The model under review builds one solid part; all positions refer to its coordinate system, in mm. A direction names the side the tool comes from. Coordinates: 2 decimals unless noted, no trailing zeros. Loops run counter-clockwise (first coordinate to the right, second up) from the corner with the lowest first, then second, coordinate; pieces in that order, holes last. Notation, with made-up numbers: M 66.25,33.5 L 125.25,33.5 A16 cw 125.25,51.5 Z; hole C 28.25,85.25 d4. An arc over 180 degrees is marked long. Return JSON: item names as keys, results as strings.
```python
from build123d import *

# Parameters (mm, degrees)
PAD_DEPTH       = 10.5
CHAMFER001_SIZE = 1
SKETCH017_R     = 1.6
POCKET010_DEPTH = 12
SKETCH018_R     = 1.95
POCKET011_DEPTH = 5
FILLET001_R     = 5
CHAMFER002_SIZE = 1
CHAMFER003_SIZE = 2.5


with BuildPart() as part:
    # Sketch016 → Pad (new body)
    with BuildSketch(Plane.XY):
        with BuildLine():
            Line((-12.5, 0), (-12.5, 10.25))
            Line((-12.5, 10.25), (-25.5, 10.25))
            Line((-25.5, 10.25), (-25.5, -26))
            Line((-25.5, -26), (25.3, -26))
            ThreePointArc((25.3, -26), (38.735029, -20.435029), (44.3, -7))
            Line((44.3, -7), (25.3, -7))
            Line((25.3, -7), (25.3, -12.5))
            Line((25.3, -12.5), (0, -12.5))
            ThreePointArc((-12.5, 0), (-8.838835, -8.838835), (0, -12.5))
        make_face()
    extrude(amount=PAD_DEPTH)

    # Chamfer001
    chamfer001_edges = [part.edges().sort_by_distance(p)[0] for p in [
        (44.3, -7, 5.25),
    ]]
    chamfer(chamfer001_edges, length=CHAMFER001_SIZE)

    # Sketch017 (on Face7 of Chamfer001) → Pocket010 (cut)
    with BuildSketch(Plane(origin=(-25.5, 0, 0), x_dir=(0, -1, 0), z_dir=(-1, 0, 0))):
        with Locations((-5.75, 3.7)):
            Circle(SKETCH017_R)
        with Locations((21.5, 3.7)):
            Circle(SKETCH017_R)
    extrude(amount=-POCKET010_DEPTH, mode=Mode.SUBTRACT)

    # Sketch018 (on Face7 of Pocket010) → Pocket011 (cut)
    with BuildSketch(Plane(origin=(-25.5, 0, 0), x_dir=(0, -1, 0), z_dir=(-1, 0, 0))):
        with Locations((-5.75, 3.7)):
            Circle(SKETCH018_R)
        with Locations((21.5, 3.7)):
            Circle(SKETCH018_R)
    extrude(amount=-POCKET011_DEPTH, mode=Mode.SUBTRACT)

    # Fillet001
    fillet001_edges = [part.edges().sort_by_distance(p)[0] for p in [
        (-12.5, 10.25, 5.25),
    ]]
    fillet(fillet001_edges, radius=FILLET001_R)

    # Chamfer002
    chamfer002_edges = [part.edges().sort_by_distance(p)[0] for p in [
        (-21.5, 10.25, 10.5),
        (-0.1, -26, 10.5),
        (-13.964466, 8.785534, 10.5),
        (-12.5, 2.625, 10.5),
        (-8.838835, -8.838835, 10.5),
        (38.376823, -20.783929, 10.5),
        (43.786842, -7.499827, 10.5),
        (34.3, -7, 10.5),
        (25.3, -9.75, 10.5),
        (12.65, -12.5, 10.5),
    ]]
    chamfer(chamfer002_edges, length=CHAMFER002_SIZE)

    # Chamfer003
    chamfer003_edges = [part.edges().sort_by_distance(p)[0] for p in [
        (-21.5, 10.25, 0),
        (-0.1, -26, 0),
    ]]
    chamfer(chamfer003_edges, length=CHAMFER003_SIZE)


with BuildPart() as part_1:
    # Body004 placement: moved
    add(part.part.moved(Location((0, 0, 6.5))))


solid = part_1.part
```
1. To check wall thickness, follow line 1 (Z direction, x = -24.35, y = 5.75); line 2 (Y direction, x = 17, z = 10.5); line 3 (X direction, y = 4.5, z = 9.75). State the ranges of each line that lie inside material, in increasing order.
Check values:
{"line 1": "6.5 to 8.25, 12.15 to 17", "line 2": "-26 to -12.5", "line 3": "-13.5 to -12.5"}
2. Add section B-B on x = 23.5. Give the boundary of the cut face in (y, z).
Check values:
{"outline": "M -26,9 L -23.5,6.5 L -15,6.5 L -12.5,9 L -12.5,16 L -13.5,17 L -25,17 L -26,16 Z"}
3. The part is to be moulded in two halves that separate along X. For faces 1 (the face through (37.1, -19.1, 6.9)), 2 (the face through (-8.935, -8.741, 12.451)), 3 (the face through (-8.86, -9.06, 16.17)), 4 (the face through (-17.05, -21.15, 8.64)), say which applies: released by +X, released by -X, zero draft, split by the parting line, or undercut.
Check values:
{"face 1": "released by +X", "face 2": "undercut", "face 3": "undercut", "face 4": "zero draft"}
4. Machinability: for faces 5 (the face through (-23.035, 7.698, 10.286)), 6 (the face through (13, -12.5, 12)), 7 (the face through (38.23, -20.92, 12.45)), 8 (the face through (-13.8, 2.6, 7.7)), 9 (the face through (-9.24, -9.44, 8.29)), which of the approach directions +Z, -Z, +X, -X, +Y, -Y give a long, thin tool a straight path to every point of the face, cutting with its end or side? Answer none if there is none.
Check values:
{"face 5": "-X", "face 6": "+Z, -Z, +Y", "face 7": "+Z, -Z, +X, -Y", "face 8": "-Z, +X, +Y", "face 9": "-Z, +Y"}
5. Add section C-C on z = 14. Give the boundary of the cut face in (x, y).
Check values:
{"outline": "M -25.5,-26 L 25.3,-26 A19 ccw 44.27,-8 L 43.3,-7 L 25.3,-7 L 25.3,-12.5 L 0,-12.5 A12.5 cw -12.5,0 L -12.5,5.25 A5 ccw -17.5,10.25 L -25.5,10.25 Z"}
6. Insertion check: pin 1 Ø5.5 at (x, z) = (12.5, 12.5) entering from +Y; pin 2 Ø2 at (x, z) = (35, 14.5) entering from -Y; pin 3 Ø2.5 at (y, z) = (-21.5, 10.2) entering from -X. Each pin has a flat end and moves straight along its axis. Give the tip position at first contact, or say it passes through.
Check values:
{"pin 1": "y = -12.5", "pin 2": "y = -23.89", "pin 3": "x = -13.5"}
7. Add section A-A on z = 10.2. Give the boundary of the cut face in (x, y).
Check values:
{"outline": "M -25.5,-26 L 25.3,-26 A19 ccw 44.27,-8 L 43.3,-7 L 25.3,-7 L 25.3,-12.5 L 0,-12.5 A12.5 cw -12.5,0 L -12.5,5.25 A5 ccw -17.5,10.25 L -25.5,10.25 L -25.5,7.7 L -20.5,7.7 L -20.5,7.35 L -13.5,7.35 L -13.5,4.15 L -20.5,4.15 L -20.5,3.8 L -25.5,3.8 L -25.5,-19.55 L -20.5,-19.55 L -20.5,-19.9 L -13.5,-19.9 L -13.5,-23.1 L -20.5,-23.1 L -20.5,-23.45 L -25.5,-23.45 Z"}
